```python
from build123d import *

# Parameters (mm, degrees)
SKETCH1_R           = 20
BOSS_EXTRUDE1_DEPTH = 10
SKETCH2_R           = 18.5
BOSS_EXTRUDE2_DEPTH = 11
SKETCH3_R           = 17
BOSS_EXTRUDE3_DEPTH = 6
SKETCH4_R           = 11
BOSS_EXTRUDE4_DEPTH = 25
FILLET1_R           = 1


with BuildPart() as part:
    # Sketch1 → Boss-Extrude1 (new body)
    with BuildSketch(Plane.XY):
        Circle(SKETCH1_R)
    extrude(amount=BOSS_EXTRUDE1_DEPTH)

    # Sketch2 → Boss-Extrude2 (add)
    with BuildSketch(Plane.XY.offset(10)):
        Circle(SKETCH2_R)
    extrude(amount=BOSS_EXTRUDE2_DEPTH)

    # Sketch3 → Boss-Extrude3 (add)
    with BuildSketch(Plane.XY.offset(21)):
        Circle(SKETCH3_R)
    extrude(amount=BOSS_EXTRUDE3_DEPTH)

    # Sketch4 → Boss-Extrude4 (add)
    with BuildSketch(Plane.XY.offset(27)):
        Circle(SKETCH4_R)
    extrude(amount=BOSS_EXTRUDE4_DEPTH)

    # Fillet1
    fillet1_edges = [part.edges().sort_by_distance(p)[0] for p in [
        (-20, 0, 0),
        (-18.5, 0, 21),
    ]]
    fillet(fillet1_edges, radius=FILLET1_R)


solid = part.part
```
Can you work these out from the model? Positions are in its coordinate system, mm. A direction names the side the tool comes from. Round coordinates to 2 decimals unless told otherwise and drop trailing zeros. Loops run counter-clockwise (first coordinate to the right, second up) from the corner with the lowest first, then second, coordinate; pieces in that order, holes last. Notation, with made-up numbers: M 7.5,-28.5 L 20.5,-28.5 A33 cw 20.5,-0.5 Z; hole C 64,69 d3. An arc over 180 degrees is marked long. Answer as a JSON object with one key per item and string values. Group by question number.
Q1. Please list where these lines run through material, in increasing order: L1, parallel to Z at x = -16.5, y = -1; L2, parallel to Y at x = 0, z = 36.5; L3, parallel to X at y = 17, z = 17.5.
Q2. Imagine slicing it at D-D, the plane z = 38. Please give me the cut outline in (x, y).
Q3. On a 3-axis mill with a long thin cutter (end or side, diameter ignored), from which of +Z, -Z, +X, -X, +Y, -Y can I reach the whole of each face in a straight line? I mean faces 4 (the flat face through (0, 0, 52)), 5 (the cylindrical face through (-2.38, -10.74, 39.33)). Say none if no direction works.
Q4. Imagine slicing it at A-A, the plane y = 0. Please give me the cut outline in (x, z).
Q5. Will these pins go through, and if not, where does the flat tip stop? pin 1 (6 mm diameter, centred on y = -7, z = 38, fed in from +X); pin 2 (4 mm diameter, centred on y = -11, z = 45.5, fed in from -X); pin 3 (2 mm diameter, centred on x = 3, z = 46.5, fed in from -Y).
Q6. We'd pull the mould along Z, two halves only. Please class faces 1 (the flat face through (0, 0, 0)), 2 (the flat face through (4, -11, 27)), 3 (the cylindrical face through (-4.01, -18.06, 14.93)): +Z half, -Z half, draft (parallel to the pull), parting line (faces both ways), or undercut.
Q7. Imagine slicing it at C-C, the plane z = 15. Please give me the cut outline in (x, y).
Findings:
{
 "1": {"L1": "z = 0 to 27", "L2": "y = -11 to 11", "L3": "x = -7.3 to 7.3"},
 "2": {"outline": "C 0,0 d22"},
 "3": {"face 4": "+Z, +X, -X, +Y, -Y", "face 5": "+Z"},
 "4": {"outline": "M -20,1 A1 ccw -19,0 L 19,0 A1 ccw 20,1 L 20,10 L 18.5,10 L 18.5,20 A1 ccw 17.5,21 L 17,21 L 17,27 L 11,27 L 11,52 L -11,52 L -11,27 L -17,27 L -17,21 L -17.5,21 A1 ccw -18.5,20 L -18.5,10 L -20,10 Z"},
 "5": {"pin 1": "stops at x = 10.25", "pin 2": "stops at x = -6.32", "pin 3": "stops at y = -10.82"},
 "6": {"face 1": "-Z half", "face 2": "+Z half", "face 3": "draft"},
 "7": {"outline": "C 0,0 d37"}
}
